CAD build for the part. Positions are in the model's coordinates, mm. A direction names the side the tool comes from. Coordinates: 2 decimals unless noted, no trailing zeros. Order: outer loops, then holes, each group sorted by start corner. A loop starts at its lowest first (then second) coordinate and runs counter-clockwise, first axis right, second up. Notation, with made-up numbers: M 56.25,64.5 L 103.25,64.5 A29 cw 103.25,96.5 Z; hole C -37,50.5 d9. An arc over 180 degrees is marked long. One line per item, written item: value.
from build123d import *

# Parameters (mm, degrees)
ESQUISSE4_R        = 23.8
BOSS_EXTRU_2_DEPTH = 19.1
ESQUISSE8_R        = 12.5
BOSS_EXTRU_3_DEPTH = 25.4
ESQUISSE9_R        = 23.8
BOSS_EXTRU_4_DEPTH = 10


with BuildPart() as part:
    # Esquisse3 → Révolution1 (revolve)
    with BuildSketch(Plane.XY):
        Polygon((0, 0), (0, 39.35), (-12.7, 39.35), (-12.7, 37.65), (-485.5, 37.65), (-485.5, 0), align=None)
    revolve(axis=Axis((-619.271971496, 0, 0), (1, 0, 0)))

    # Esquisse4 → Boss.-Extru.2 (add)
    with BuildSketch(Plane.ZY.offset(485.5)):
        Circle(ESQUISSE4_R)
    extrude(amount=BOSS_EXTRU_2_DEPTH)

    # Esquisse8 → Boss.-Extru.3 (add)
    with BuildSketch(Plane.ZY.offset(504.6)):
        Circle(ESQUISSE8_R)
    extrude(amount=BOSS_EXTRU_3_DEPTH)

    # Esquisse9 → Boss.-Extru.4 (add)
    with BuildSketch(Plane(origin=(0, 0, 0), x_dir=(0, 0, -1), z_dir=(1, 0, 0))):
        Circle(ESQUISSE9_R)
    extrude(amount=BOSS_EXTRU_4_DEPTH)


solid = part.part
Q1. Which spindle directions (+Z, -Z, +X, -X, +Y, -Y) get a long thin tool onto all of the face, cutting with end or side? Do faces 1 (the face through (-504.6, -10, 10)), 2 (the face through (4.93, 16.085, 17.542)), 3 (the face through (-530, 0, 0)). Say none if no direction does.
Recorded:
face 1: -X
face 2: +X
face 3: +Z, -Z, -X, +Y, -Y
Q2. Pin check, flat tips, straight feed: pin 1 Ø5 at (x, y) = (-412.5, 18.5) entering from +Z; pin 2 Ø4 at (x, y) = (-200, 28) entering from -Z; pin 3 Ø4 at (y, z) = (-1, 19) entering from -X. Stop position of each tip, or through.
Recorded:
pin 1: stops at z = 34.08
pin 2: stops at z = -27.23
pin 3: stops at x = -504.6
Q3. Drill centre lines: line 1 along X through (y, z) = (-32, -7); line 2 along Z through (x, y) = (-486, -2); line 3 along X through (y, z) = (-2, -23.5). Where is each one in solid material? Low to high.
Recorded:
line 1: x = -485.5 to 0
line 2: z = -23.72 to 23.72
line 3: x = -504.6 to 10
Q4. Slice it at C-C (x = -496.5). List the corners of the cut face in (y, z).
Recorded:
outline: C 0,0 d47.6
Q5. Slice it at A-A (y = 0). List the corners of the cut face in (x, z).
Recorded:
outline: M -530,-12.5 L -504.6,-12.5 L -504.6,-23.8 L -485.5,-23.8 L -485.5,-37.65 L -12.7,-37.65 L -12.7,-39.35 L 0,-39.35 L 0,-23.8 L 10,-23.8 L 10,23.8 L 0,23.8 L 0,39.35 L -12.7,39.35 L -12.7,37.65 L -485.5,37.65 L -485.5,23.8 L -504.6,23.8 L -504.6,12.5 L -530,12.5 Z
Q6. Slice it at D-D (x = -440.5). List the corners of the cut face in (y, z).
Recorded:
outline: C 0,0 d75.3
